```python
from build123d import *

# Parameters (mm, degrees)
F1_DEPTH = 5.9944
F0_R     = 13.0048
F2_DEPTH = 20.0025
F0_R_2   = 5.371097
F0_R_3   = 5.9944
F3_DEPTH = 13.0048


with BuildPart() as f1:
    # F0 (on Front) → F1 (new body, symmetric)
    with BuildSketch(Plane.XZ):
        with BuildLine():
            ThreePointArc((-72.526456, -36.31248), (-60.524956, -24.31098), (-48.523456, -36.31248))
            ThreePointArc((-48.523456, -36.31248), (-49.624469, -41.333973), (-52.725496, -45.434126))
            Line((-52.725496, -45.434126), (1.699654, 1.102078))
            Line((1.699654, 1.102078), (12.083406, 10.143629))
            ThreePointArc((12.083406, 10.143629), (18.620412, 13.016223), (25.631266, 11.662642))
            ThreePointArc((25.631266, 11.662642), (12.476738, 34.549967), (27.173551, 56.478828))
            Line((27.173551, 56.478828), (-65.465781, 14.629807))
            ThreePointArc((-65.465781, 14.629807), (-54.015782, 13.775509), (-48.523456, 3.69252))
            ThreePointArc((-48.523456, 3.69252), (-60.524956, -8.30898), (-72.526456, 3.69252))
            Line((-72.526456, 3.69252), (-72.526456, -36.31248))
        make_face()
    extrude(amount=F1_DEPTH, both=True)

    # F0 (on Front) → F2 (join, symmetric)
    with BuildSketch(Plane.XZ):
        with BuildLine():
            ThreePointArc((62.474544, 33.68992), (51.030745, 54.698814), (27.173551, 56.478828))
            ThreePointArc((27.173551, 56.478828), (12.476738, 34.549967), (25.631266, 11.662642))
            ThreePointArc((25.631266, 11.662642), (50.300158, 12.226998), (62.474544, 33.68992))
        make_face()
        with Locations((37.468244, 33.68992)):
            Circle(F0_R, mode=Mode.SUBTRACT)
    extrude(amount=F2_DEPTH, both=True)

    # F0 (on Front) → F3 (join, symmetric)
    with BuildSketch(Plane.XZ):
        with BuildLine():
            ThreePointArc((-65.465781, 14.629807), (-70.607945, 10.201694), (-72.526456, 3.69252))
            ThreePointArc((-72.526456, 3.69252), (-60.524956, -8.30898), (-48.523456, 3.69252))
            ThreePointArc((-48.523456, 3.69252), (-54.015782, 13.775509), (-65.465781, 14.629807))
        make_face()
        with Locations((-60.524956, 3.69252)):
            Circle(F0_R_2, mode=Mode.SUBTRACT)
        with BuildLine():
            ThreePointArc((-52.725496, -45.434126), (-49.624469, -41.333973), (-48.523456, -36.31248))
            ThreePointArc((-48.523456, -36.31248), (-60.524956, -24.31098), (-72.526456, -36.31248))
            ThreePointArc((-72.526456, -36.31248), (-65.546449, -47.212966), (-52.725496, -45.434126))
        make_face()
        with Locations((-60.524956, -36.31248)):
            Circle(F0_R_3, mode=Mode.SUBTRACT)
    extrude(amount=F3_DEPTH, both=True)


solid = f1.part
```
The listing builds one solid part. Answer for the finished solid, in the listing's coordinates (mm). A direction names the side the tool comes from. Round coordinates to 2 decimals unless told otherwise and drop trailing zeros. Loops run counter-clockwise (first coordinate to the right, second up) from the corner with the lowest first, then second, coordinate; pieces in that order, holes last. Notation, with made-up numbers: (4.5, 4.25) -> (57.5, 4.25) arc R7 ccw to (57.5, 13.25) -> close; hole circle Ø8 at (46.5, -12). An arc over 180 degrees is marked (long way). Use one line per item in the form item = value.
1. The part is cut by section B-B on z = -40.5. Determine the outline of the cut face in (x, y), and give its area (3 significant figures).
Answer key:
outline = (-71.77, -13) -> (-64.81, -13) -> (-64.81, 13) -> (-71.77, 13) -> close; (-56.24, -13) -> (-49.28, -13) -> (-49.28, -5.99) -> (-46.95, -5.99) -> (-46.95, 5.99) -> (-49.28, 5.99) -> (-49.28, 13) -> (-56.24, 13) -> close
area = 390 mm²
2. The part is cut by section A-A on y = -9. Determine the outline of the cut face in (x, z), and give its area (3 significant figures).
Answer key:
outline = (-72.53, 3.69) arc R12 ccw (long way) to (-65.47, 14.63) arc R12 ccw to start; (-52.73, -45.43) arc R12 ccw to (-48.52, -36.31) arc R12 ccw (long way) to start; (25.63, 11.66) arc R25.01 ccw (long way) to (27.17, 56.48) arc R25.01 ccw to start; hole circle Ø11.99 at (-60.52, -36.31); hole circle Ø10.74 at (-60.52, 3.69); hole circle Ø26.01 at (37.47, 33.69)
area = 2,130 mm²
3. Find the intervals of material crossed by probe 1 along X at (y, z) = (-10.5, -40); probe 2 along Y at (x, z) = (-40.5, 2); probe 3 along X at (y, z) = (12.5, 44), in increasing order. Write a range as [from, to].
Answer key:
probe_1 = [-71.95, -65.25], [-55.8, -49.1]
probe_2 = [-5.99, 5.99]
probe_3 = [14.69, 29.54], [45.39, 60.25]
4. A tool of negligible diameter and unlimited length cuts with its end or side. For faces 1 (the flat face through (-18.498, -0.084, 35.847)), 2 (the flat face through (-55, 13.005, 1)), 3 (the flat face through (-55, -13.005, 1)), from which of +Z, -Z, +X, -X, +Y, -Y can it reach the whole face along a straight path? Write none if from no direction.
Answer key:
face_1 = +Z, -X, +Y, -Y
face_2 = +Z, -Z, -X, +Y
face_3 = +Z, -Z, -X, -Y
5. The part is cut by section C-C on y = 3.5. Determine the outline of the cut face in (x, z).
Answer key:
outline = (-72.53, -36.31) arc R12 ccw to (-52.73, -45.43) -> (1.7, 1.1) -> (12.08, 10.14) arc R11.99 cw to (25.63, 11.66) arc R25.01 ccw (long way) to (27.17, 56.48) -> (-65.47, 14.63) arc R12 ccw to (-72.53, 3.69) -> close; hole circle Ø11.99 at (-60.52, -36.31); hole circle Ø10.74 at (-60.52, 3.69); hole circle Ø26.01 at (37.47, 33.69)
6. Flat-ended cylindrical pins translate along their axes: pin 1 Ø3 at (y, z) = (-4.5, 18) entering from +X; pin 2 Ø1.5 at (x, y) = (1.5, -4.5) entering from -Z; pin 3 Ø2 at (x, z) = (-15.5, -17.5) entering from +Y; pin 4 Ø7 at (x, z) = (-55.5, -37) entering from +Y. Find the tip coordinate at first contact, or state that the pin passes through.
Answer key:
pin_1 = 58.06
pin_2 = 0.29
pin_3 = through
pin_4 = 13
7. For a pull along Z with two mould halves and no side action, classify faces 4 (the cylindrical face through (-61.824, 0.182, -42.164)), 5 (the flat face through (-25.89, -0.08, -22.49)), 6 (the flat face through (48, -20.002, 23)) as released by +Z, released by -Z, zero draft, split by the parting line, or undercut.
Answer key:
face_4 = undercut
face_5 = released by -Z
face_6 = zero draft
8. The part is cut by section D-D on y = 15. Determine the outline of the cut face in (x, z).
Answer key:
outline = (25.63, 11.66) arc R25.01 ccw (long way) to (27.17, 56.48) arc R25.01 ccw to start; hole circle Ø26.01 at (37.47, 33.69)
